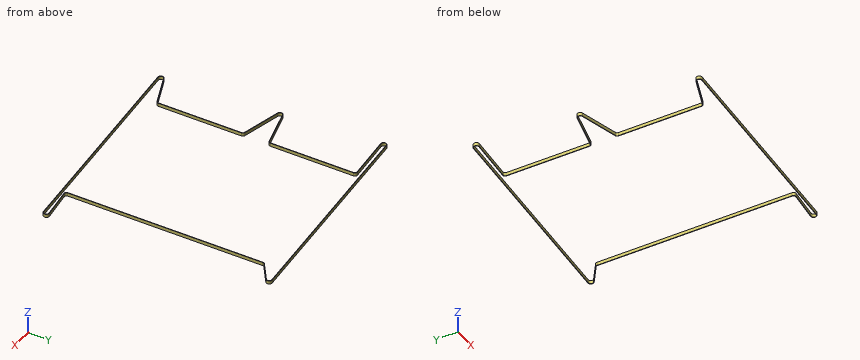
from build123d import *

# Parameters (mm, degrees)
EXTRUDE_1_DEPTH = 4.5


with BuildPart() as part:
    # Эскиз2 → Вытянуть-Тонкостенный1 (new, symmetric)
    with BuildSketch(Plane.XY):
        with BuildLine():
            Line((5.3, 230), (5.3, 0))
            ThreePointArc((5.3, 0), (4.183794955, -3.253591827), (1.305335933, -5.136740027))
            Line((1.305335933, -5.136740027), (-104.994947369, -32.149510525))
            ThreePointArc((-104.994947369, -32.149510525), (-111.1, -40), (-104.994947369, -47.850489475))
            Line((-104.994947369, -47.850489475), (1.305335933, -74.863259973))
            ThreePointArc((1.305335933, -74.863259973), (4.183794955, -76.746408173), (5.3, -80))
            Line((5.3, -80), (5.3, -310))
            ThreePointArc((5.3, -310), (4.379504294, -312.98495262), (1.937757682, -314.933061439))
            Line((1.937757682, -314.933061439), (-85.961478722, -349.460792895))
            ThreePointArc((-85.961478722, -349.460792895), (-90.898089189, -358.797272144), (-82.407590787, -365.078307454))
            Line((-82.407590787, -365.078307454), (517.592409213, -321.078307454))
            ThreePointArc((517.592409213, -321.078307454), (525.062194527, -312.218322694), (516.029484483, -304.958352182))
            Line((516.029484483, -304.958352182), (430.655423427, -315.261818943))
            ThreePointArc((430.655423427, -315.261818943), (426.504406414, -313.965832319), (424.720394755, -310))
            Line((424.720394755, -310), (424.720394755, 230))
            ThreePointArc((424.720394755, 230), (425.310455419, 232.430323322), (426.949251906, 234.319500156))
            Line((426.949251906, 234.319500156), (477.693633412, 270.398499762))
            ThreePointArc((477.693633412, 270.398499762), (480.620970965, 279.744230593), (472.407590787, 285.078307454))
            Line((472.407590787, 285.078307454), (-127.592409213, 241.078307454))
            ThreePointArc((-127.592409213, 241.078307454), (-135.075604128, 232.371813747), (-126.336049032, 224.927257646))
            Line((-126.336049032, 224.927257646), (-0.434437053, 235.28216475))
            ThreePointArc((-0.434437053, 235.28216475), (3.590785681, 233.898237831), (5.3, 230))
        make_face()
        with BuildLine():
            Line((6.7, 230), (6.7, 0))
            ThreePointArc((6.7, 0), (5.288948339, -4.113031178), (1.650141651, -6.493614751))
            Line((1.650141651, -6.493614751), (-104.650141651, -33.506385249))
            ThreePointArc((-104.650141651, -33.506385249), (-109.7, -40), (-104.650141651, -46.493614751))
            Line((-104.650141651, -46.493614751), (1.650141651, -73.506385249))
            ThreePointArc((1.650141651, -73.506385249), (5.288948339, -75.886968822), (6.7, -80))
            Line((6.7, -80), (6.7, -310))
            ThreePointArc((6.7, -310), (5.536354485, -313.77343067), (2.449618202, -316.236134272))
            Line((2.449618202, -316.236134272), (-85.449618202, -350.763865728))
            ThreePointArc((-85.449618202, -350.763865728), (-89.532987354, -358.486632515), (-82.509982503, -363.682056783))
            Line((-82.509982503, -363.682056783), (517.490017497, -319.682056783))
            ThreePointArc((517.490017497, -319.682056783), (523.668728806, -312.353427414), (516.197227906, -306.34826662))
            Line((516.197227906, -306.34826662), (430.82316685, -316.65173338))
            ThreePointArc((430.82316685, -316.65173338), (425.575654776, -315.013410667), (423.320394755, -310))
            Line((423.320394755, -310), (423.320394755, 230))
            ThreePointArc((423.320394755, 230), (424.0663205, 233.07229552), (426.138006625, 235.460500197))
            Line((426.138006625, 235.460500197), (476.882388131, 271.539499803))
            ThreePointArc((476.882388131, 271.539499803), (479.303766107, 279.269919132), (472.509982503, 283.682056783))
            Line((472.509982503, 283.682056783), (-127.490017497, 239.682056783))
            ThreePointArc((-127.490017497, 239.682056783), (-133.679820698, 232.480389148), (-126.450805989, 226.322546448))
            Line((-126.450805989, 226.322546448), (-0.549194011, 236.677453552))
            ThreePointArc((-0.549194011, 236.677453552), (4.539295107, 234.927961032), (6.7, 230))
        make_face(mode=Mode.SUBTRACT)
    extrude(amount=EXTRUDE_1_DEPTH, both=True)


solid = part.part
Could you check a few things on this model? Use its own coordinates, in mm. Round coordinates to 2 decimals unless told otherwise and drop trailing zeros. Write each loop counter-clockwise with the first axis right and the second up, starting at its lowest first coordinate (ties: lowest second). Pieces come first, ordered by that corner, then holes. Notation, with made-up numbers: (15, -32.5) - (38, -32.5) arc R29 ccw to (38, 0.5) - close; hole circle Ø3 at (58.5, 82). An arc over 180 degrees is marked (long way). Use a Markdown table: item, result.
Q1. I want a section at A-A (y = 92). List the corners of the cut face in (x, z) for me, plus the area to 3 significant figures.
Output values:
| item | result |
|---|---|
| outline | (5.3, -4.5) - (6.7, -4.5) - (6.7, 4.5) - (5.3, 4.5) - close; (423.32, -4.5) - (424.72, -4.5) - (424.72, 4.5) - (423.32, 4.5) - close |
| area | 25.2 mm2 |
Q2. For pin 1 (1.5 mm diameter, centred on x = -19, z = -3.5, fed in from +Y); pin 2 (4.5 mm diameter, centred on y = 29.5, z = -1, fed in from -X); pin 3 (3 mm diameter, centred on y = -8.5, z = 3, fed in from +X), each with a flat end and sliding along its axis, tell me the tip position at first contact or that it passes through.
Output values:
| item | result |
|---|---|
| pin 1 | y = 249.1 |
| pin 2 | x = 5.3 |
| pin 3 | x = 424.72 |
Q3. Please list where these lines run through material, in increasing order: L1, parallel to X at y = 211, z = -2; L2, parallel to Y at x = -76, z = 2; L3, parallel to Y at x = -21.5, z = 0.5.
Output values:
| item | result |
|---|---|
| L1 | 5.3 to 6.7, 423.32 to 424.72 |
| L2 | -364.61 to -363.2, -347.05 to -345.55, -55.22 to -53.77, -26.23 to -24.78, 229.07 to 230.47, 243.46 to 244.86 |
| L3 | -360.61 to -359.21, -325.64 to -324.14, -69.07 to -67.62, -12.38 to -10.93, 233.55 to 234.95, 247.45 to 248.86 |
Q4. I want a section at B-B (x = 391.5). List the corners of the cut face in (y, z) for me.
Output values:
| item | result |
|---|---|
| outline | (-330.33, -4.5) - (-328.92, -4.5) - (-328.92, 4.5) - (-330.33, 4.5) - close; (277.74, -4.5) - (279.15, -4.5) - (279.15, 4.5) - (277.74, 4.5) - close |
